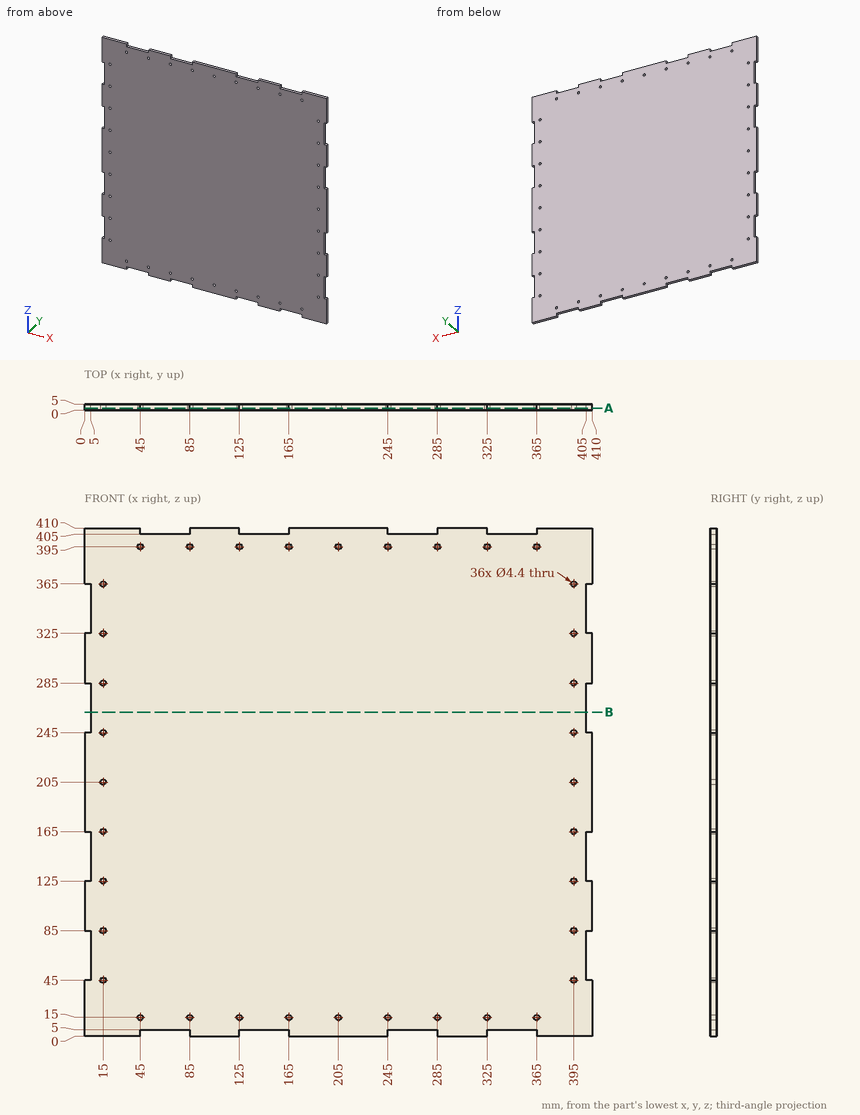
Can you work these out from the drawing? Everything is in mm from the part's minimum corner. Round coordinates to 2 decimals unless told otherwise and drop trailing zeros. Write each loop counter-clockwise with the first axis right and the second up, starting at its lowest first coordinate (ties: lowest second). Pieces come first, ordered by that corner, then holes. Notation, with made-up numbers: (7, 19) - (57, 19) arc R15 ccw to (57, 45) - close; hole circle Ø7 at (29.25, 33). An arc over 180 degrees is marked (long way). Use a Markdown table: item, result.
Q1. Please list where these lines run through material, in increasing order: L1, parallel to Z at x = 364.5, y = 1.2; L2, parallel to Z at x = 269.5, y = 2.75.
Output values:
| item | result |
|---|---|
| L1 | 5 to 12.86, 17.14 to 392.86, 397.14 to 405 |
| L2 | 5 to 405 |
Q2. I want a section at B-B (z = 261.5). List the corners of the cut face in (x, y) for me, plus the area to 3 significant figures.
Output values:
| item | result |
|---|---|
| outline | (5, 0) - (405, 0) - (405, 5) - (5, 5) - close |
| area | 2,000 mm2 |
Q3. I want a section at A-A (y = 1.6). Count the separate pieces of the cut face and the enclosed holes in it, plus the area to 3 significant figures.
Output values:
| item | result |
|---|---|
| separate pieces | 1 |
| enclosed holes | 36 |
| area | 164,000 mm2 |
Q4. For pin 1 (4 mm diameter, centred on x = 15, z = 85, fed in from +Y); pin 2 (2.5 mm diameter, centred on y = 3.5, z = 271.5, fed in from -X), each with a flat end and sliding along its axis, tell me the tip position at first contact or that it passes through.
Output values:
| item | result |
|---|---|
| pin 1 | through |
| pin 2 | x = 5 |
